```python
from build123d import *

# Parameters (mm, degrees)
BOSS_EXTRUDE1_DEPTH     = 127
SKETCH3_W               = 5
SKETCH3_H               = 42.3
BOSS_EXTRUDE2_DEPTH     = 42.3
SKETCH4_R               = 1.7
CUT_EXTRUDE1_DEPTH      = 5
CUT_EXTRUDE7_DEPTH      = 161.690696682
CUT_EXTRUDE7_DEPTH_BACK = 161.690696682
SKETCH5_R               = 1.7
SKETCH8_R               = 3.2
CUT_EXTRUDE8_DEPTH      = 2
SKETCH10_W              = 20
SKETCH10_H              = 10
BOSS_EXTRUDE3_DEPTH     = 35
FILLET3_R               = 5
SKETCH12_R              = 1.7
CUT_EXTRUDE9_DEPTH      = 35
RIB47_START             = -2
RIB47_DEPTH             = 2
FILLET7_R               = 5
FILLET8_R               = 2
SKETCH18_W              = 6.4
SKETCH18_H              = 20
CUT_EXTRUDE10_DEPTH     = 9
SKETCH19_W              = 5
SKETCH19_H              = 18
CUT_EXTRUDE11_DEPTH     = 4


# Read off the part's stored shape, not the designer's step: Rib47
with BuildPart() as part:
    # Sketch2 → Boss-Extrude1 (new body)
    with BuildSketch(Plane(origin=(0, 0, 0), x_dir=(1, 0, 0), z_dir=(0, 1, 0))):
        with BuildLine():
            Line((-5.331538291, 0), (-3, -5))
            Line((-3, -5), (-47, -5))
            Line((-47, -5), (-44.668461709, 0))
            Line((-44.668461709, 0), (-55.331538291, 0))
            Line((-55.331538291, 0), (-53, -5))
            Line((-53, -5), (-81.4, -5))
            ThreePointArc((-81.4, -5), (-86.703300859, -7.196699141), (-88.9, -12.5))
            Line((-88.9, -12.5), (-88.9, -17.5))
            ThreePointArc((-88.9, -17.5), (-86.703300859, -22.803300859), (-81.4, -25))
            Line((-81.4, -25), (81.4, -25))
            ThreePointArc((81.4, -25), (86.703300859, -22.803300859), (88.9, -17.5))
            Line((88.9, -17.5), (88.9, -12.5))
            ThreePointArc((88.9, -12.5), (86.703300859, -7.196699141), (81.4, -5))
            Line((81.4, -5), (53, -5))
            Line((53, -5), (55.331538291, 0))
            Line((55.331538291, 0), (44.668461709, 0))
            Line((44.668461709, 0), (47, -5))
            Line((47, -5), (3, -5))
            Line((3, -5), (5.331538291, 0))
            Line((5.331538291, 0), (-5.331538291, 0))
        make_face()
    extrude(amount=BOSS_EXTRUDE1_DEPTH)

    # Sketch3 → Boss-Extrude2 (add)
    with BuildSketch(Plane.XY.offset(25)):
        with Locations((-13.06, 55.018873206)):
            Rectangle(SKETCH3_W, SKETCH3_H)
    extrude(amount=BOSS_EXTRUDE2_DEPTH)

    # Sketch4 → Cut-Extrude1 (cut)
    with BuildSketch(Plane(origin=(-10.56, 0, 0), x_dir=(0, 0, -1), z_dir=(1, 0, 0))):
        with BuildLine():
            ThreePointArc((-34.95, 55.018873206), (-46.15, 66.218873206), (-57.35, 55.018873206))
            Line((-57.35, 55.018873206), (-34.95, 55.018873206))
        make_face()
        with BuildLine():
            Line((-34.95, 55.018873206), (-57.35, 55.018873206))
            ThreePointArc((-57.35, 55.018873206), (-46.15, 43.818873206), (-34.95, 55.018873206))
        make_face()
        with Locations((-61.65, 70.518873206)):
            Circle(SKETCH4_R)
        with Locations((-30.65, 70.518873206)):
            Circle(SKETCH4_R)
        with Locations((-30.65, 39.518873206)):
            Circle(SKETCH4_R)
        with Locations((-61.65, 39.518873206)):
            Circle(SKETCH4_R)
    extrude(amount=-CUT_EXTRUDE1_DEPTH, mode=Mode.SUBTRACT)

    # Sketch5 → Cut-Extrude7 (cut, two sides: drawn at the far end of the back side and taken through both)
    with BuildSketch(Plane.XY.offset(25).offset(-CUT_EXTRUDE7_DEPTH_BACK)):
        with Locations(Location((-58.65, 118.5, 0), (0, 0, 180))):
            Circle(SKETCH5_R)
        with Locations((58.65, 118.5)):
            Circle(SKETCH5_R)
        with Locations((58.65, 8.5)):
            Circle(SKETCH5_R)
        with Locations(Location((-58.65, 8.5, 0), (0, 0, 180))):
            Circle(SKETCH5_R)
    extrude(amount=CUT_EXTRUDE7_DEPTH + CUT_EXTRUDE7_DEPTH_BACK, mode=Mode.SUBTRACT)

    # Sketch8 → Cut-Extrude8 (cut)
    with BuildSketch(Plane(origin=(0, 0, 5), x_dir=(-1, 0, 0), z_dir=(0, 0, -1))):
        with Locations((-58.65, 118.5)):
            Circle(SKETCH8_R)
        with Locations((-58.65, 8.5)):
            Circle(SKETCH8_R)
        with Locations((58.65, 118.5)):
            Circle(SKETCH8_R)
        with Locations((58.65, 8.5)):
            Circle(SKETCH8_R)
    extrude(amount=-CUT_EXTRUDE8_DEPTH, mode=Mode.SUBTRACT)

    # Sketch10 → Boss-Extrude3 (add)
    with BuildSketch(Plane.XY.offset(25)):
        with Locations((0, 5)):
            Rectangle(SKETCH10_W, SKETCH10_H)
    extrude(amount=BOSS_EXTRUDE3_DEPTH)

    # Fillet3
    fillet3_edges = [part.edges().sort_by_distance(p)[0] for p in [
        (-10, 5, 60),
        (10, 5, 60),
    ]]
    fillet(fillet3_edges, radius=FILLET3_R)

    # Sketch12 → Cut-Extrude9 (cut)
    with BuildSketch(Plane(origin=(0, 10, 0), x_dir=(1, 0, 0), z_dir=(0, 1, 0))):
        with Locations(Location((0, -54, 0), (0, 0, 270))):
            Circle(SKETCH12_R)
    extrude(amount=-CUT_EXTRUDE9_DEPTH, mode=Mode.SUBTRACT)

    # Rib47 outline → Rib47 (add)
    with BuildSketch(Plane(origin=(10, 0, 0), x_dir=(0, 0, -1), z_dir=(1, 0, 0)).offset(RIB47_START)):
        Polygon((-25, 35.191123447), (-50.191123447, 10), (-25, 10), align=None)
    rib47 = extrude(amount=RIB47_DEPTH)

    # Mirror1: Rib47 across plane
    add(rib47.mirror(Plane(origin=(0, 0, 0), x_dir=(0, 0, 1), z_dir=(1, 0, 0))))

    # Fillet7
    # the kernel refuses this fillet: 5 mm, written as the material it adds along each edge
    with BuildSketch(Plane(origin=(-10, 47.691123447, 25), x_dir=(-1, 0, 0), z_dir=(0, -1, 0))) as fillet7_piece_1_section:
        with BuildLine():
            CenterArc((FILLET7_R, -FILLET7_R), FILLET7_R, 90, 90)
            Line((0, -FILLET7_R), (0, 0))
            Line((0, 0), (FILLET7_R, 0))
        make_face()
    fillet7_piece_1 = extrude(amount=47.691123447, mode=Mode.PRIVATE)
    fillet7_piece_1 = split(fillet7_piece_1, bisect_by=Plane(origin=(-11.152129269, 25.569946894, 34.621176553), z_dir=(0, -0.7071067811865476, -0.7071067811865476)), keep=Keep.TOP, mode=Mode.PRIVATE)
    add(fillet7_piece_1)
    with BuildSketch(Plane(origin=(10, 47.691123447, 25), x_dir=(0, 0, 1), z_dir=(0, -1, 0))) as fillet7_piece_2_section:
        with BuildLine():
            CenterArc((FILLET7_R, -FILLET7_R), FILLET7_R, 90, 90)
            Line((0, -FILLET7_R), (0, 0))
            Line((0, 0), (FILLET7_R, 0))
        make_face()
    fillet7_piece_2 = extrude(amount=47.691123447, mode=Mode.PRIVATE)
    fillet7_piece_2 = split(fillet7_piece_2, bisect_by=Plane(origin=(11.152129269, 25.569946894, 34.621176553), z_dir=(0, -0.7071067811865476, -0.7071067811865476)), keep=Keep.TOP, mode=Mode.PRIVATE)
    add(fillet7_piece_2)

    # Fillet8
    fillet8_edges = [part.edges().sort_by_distance(p)[0] for p in [
        (0, 10, 25),
        (8, 22.595561724, 25),
        (11.5, 35.191123447, 25),
        (-9.28, 35.191123447, 25),
        (-8, 22.595561724, 25),
    ]]
    fillet(fillet8_edges, radius=FILLET8_R)

    # Sketch18 → Cut-Extrude10 (cut)
    with BuildSketch(Plane(origin=(0, 10, 0), x_dir=(1, 0, 0), z_dir=(0, 1, 0))):
        with Locations((0, -39.517084206)):
            Rectangle(SKETCH18_W, SKETCH18_H)
    extrude(amount=-CUT_EXTRUDE10_DEPTH, mode=Mode.SUBTRACT)

    # Sketch19 → Cut-Extrude11 (cut)
    with BuildSketch(Plane(origin=(0, 1, 0), x_dir=(1, 0, 0), z_dir=(0, 1, 0))):
        with Locations((0, -40.017084206)):
            Rectangle(SKETCH19_W, SKETCH19_H)
    extrude(amount=-CUT_EXTRUDE11_DEPTH, mode=Mode.SUBTRACT)


solid = part.part
```
Check sheet for the modelled part. Datum: model origin and axes. Units: mm. A direction names the side the tool comes from. Round coordinates to 2 decimals unless told otherwise and drop trailing zeros. Loops run counter-clockwise (first coordinate to the right, second up) from the corner with the lowest first, then second, coordinate; pieces in that order, holes last. Notation, with made-up numbers: (68.5, 7.25) -> (110.5, 7.25) arc R23 ccw to (110.5, 45.25) -> close; hole circle Ø11 at (20.5, -35). An arc over 180 degrees is marked (long way). Write item = value, one per line. Start each with the question number.
1) Sectioned sample at A-A, the plane y = 97. Record the cut outline in (x, z), plus the area to 3 significant figures.
2) Sectioned sample at B-B, the plane x = 37.5. Record the cut outline in (y, z).
3) Release check for a two-part mould opening along X. For faces 1 (the flat face through (-88.9, 63, 15)), 2 (the flat face through (50, 63, 0)), 3 (the flat face through (-10.56, 64, 55)), 4 (the cylindrical face through (-55.453, 8.641, 5.986)) record: released by +X, released by -X, zero draft, split by the parting line, or undercut.
4) Thickness scan on probe 1 along X at (y, z) = (14.5, 32); probe 2 along X at (y, z) = (6, 54); probe 3 along Y at (x, z) = (-13.4, 30.65). Record the ranges inside material, lowest first.
5) Gauge pin test, flat ends, axial feed: pin 1 Ø1.5 at (x, z) = (1.5, 42) entering from -Y; pin 2 Ø14 at (x, y) = (64.5, 82) entering from -Z; pin 3 Ø4.5 at (y, z) = (6, 42.5) entering from -X; pin 4 Ø1.5 at (x, z) = (-12.5, 53) entering from +Y. Record the tip position at first contact, or that the pin passes through.
6) Set-up check for faces 5 (the flat face through (0, 63, 0)), 6 (the cylindrical face through (56.93, 121.2, 5.99)), 7 (the flat face through (-3.2, 6, 40)), 8 (the flat face through (-13, 76.169, 46)), 9 (the flat face through (10, 9, 40)): record each of +Z, -Z, +X, -X, +Y, -Y from which the full face is reachable in a straight line by a thin tool's end or side.
Results are:
q1.outline = (-88.9, 12.5) arc R7.5 ccw to (-81.4, 5) -> (-53, 5) -> (-55.33, 0) -> (-44.67, 0) -> (-47, 5) -> (-3, 5) -> (-5.33, 0) -> (5.33, 0) -> (3, 5) -> (47, 5) -> (44.67, 0) -> (55.33, 0) -> (53, 5) -> (81.4, 5) arc R7.5 ccw to (88.9, 12.5) -> (88.9, 17.5) arc R7.5 ccw to (81.4, 25) -> (-81.4, 25) arc R7.5 ccw to (-88.9, 17.5) -> close
q1.area = 3,630 mm^2
q2.outline = (0, 5) -> (127, 5) -> (127, 25) -> (0, 25) -> close
q3.face_1 = released by -X
q3.face_2 = zero draft
q3.face_3 = released by +X
q3.face_4 = undercut
q4.probe_1 = -10 to -8, 8 to 10
q4.probe_2 = -10 to -1.7, 1.7 to 10
q4.probe_3 = 33.87 to 37.82, 41.22 to 68.82, 72.22 to 76.17
q5.pin_1 = through
q5.pin_2 = 5
q5.pin_3 = -10
q5.pin_4 = 76.17
q6.face_5 = -Z, +X, -X, +Y, -Y
q6.face_6 = -Z
q6.face_7 = +Y
q6.face_8 = +Z, +X, -X, +Y
q6.face_9 = +Z, +X, +Y, -Y
